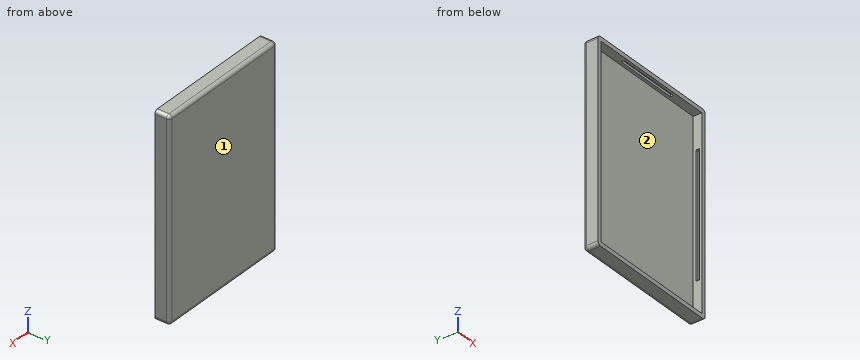
```python
from build123d import *

# Parameters (mm, degrees)
MAIN_LID_W          = 41.7
MAIN_LID_H          = 60.2
MAIN_LID_W_2        = 39.2
MAIN_LID_H_2        = 57.7
BOSS_EXTRUDE1_DEPTH = 4.5
MAIN_LID_3_W        = 39.2
MAIN_LID_3_H        = 57.7
CUT_EXTRUDE1_DEPTH  = 2.65
SKETCH2_W           = 17.05
SKETCH2_H           = 0.9
CUT_EXTRUDE2_DEPTH  = 0.75
SKETCH3_W           = 37.7
SKETCH3_H           = 1.05
CUT_EXTRUDE3_DEPTH  = 0.75
SKETCH4_W           = 19.2
SKETCH4_H           = 0.9
CUT_EXTRUDE4_DEPTH  = 0.75
FILLET1_R           = 1


with BuildPart() as part:
    # Main_Lid → Boss-Extrude1 (new body)
    # profile 1 of 2: a face of its own
    with BuildSketch(Plane(origin=(0, -69.305732589, 0), x_dir=(1, 0, 0), z_dir=(0, 1, 0))):
        with Locations((41.6, 0.1)):
            Rectangle(MAIN_LID_W, MAIN_LID_H)
        with Locations((41.6, 0.1)):
            Rectangle(MAIN_LID_W_2, MAIN_LID_H_2, mode=Mode.SUBTRACT)
    # profile 2 of 2: a face of its own
    with BuildSketch(Plane(origin=(0, -69.305732589, 0), x_dir=(1, 0, 0), z_dir=(0, 1, 0))):
        with Locations((41.6, 0.1)):
            Rectangle(MAIN_LID_W_2, MAIN_LID_H_2)
    extrude(amount=BOSS_EXTRUDE1_DEPTH)

    # Main_Lid_3 → Cut-Extrude1 (cut)
    with BuildSketch(Plane(origin=(0, -69.305732589, 0), x_dir=(1, 0, 0), z_dir=(0, 1, 0))):
        with Locations((41.6, 0.1)):
            Rectangle(MAIN_LID_3_W, MAIN_LID_3_H)
    extrude(amount=CUT_EXTRUDE1_DEPTH, mode=Mode.SUBTRACT)

    # Sketch2 → Cut-Extrude2 (cut)
    with BuildSketch(Plane.XY.offset(-28.95)):
        with Locations((49.675, -68.055732589)):
            Rectangle(SKETCH2_W, SKETCH2_H)
    extrude(amount=-CUT_EXTRUDE2_DEPTH, mode=Mode.SUBTRACT)

    # Sketch3 → Cut-Extrude3 (cut)
    with BuildSketch(Plane.ZY.offset(-61.2)):
        with Locations((-0.1, -67.980732589)):
            Rectangle(SKETCH3_W, SKETCH3_H)
    extrude(amount=-CUT_EXTRUDE3_DEPTH, mode=Mode.SUBTRACT)

    # Sketch4 → Cut-Extrude4 (cut)
    with BuildSketch(Plane(origin=(0, 0, 28.75), x_dir=(-1, 0, 0), z_dir=(0, 0, -1))):
        with Locations((-41.6, -68.055732589)):
            Rectangle(SKETCH4_W, SKETCH4_H)
    extrude(amount=-CUT_EXTRUDE4_DEPTH, mode=Mode.SUBTRACT)

    # Fillet1
    fillet1_edges = [part.edges().sort_by_distance(p)[0] for p in [
        (20.75, -67.055732589, 30),
        (41.6, -64.805732589, 30),
        (62.45, -64.805732589, -0.1),
        (41.6, -64.805732589, -30.2),
        (20.75, -64.805732589, -0.1),
        (20.75, -67.055732589, -30.2),
        (62.45, -67.055732589, -30.2),
        (62.45, -67.055732589, 30),
    ]]
    fillet(fillet1_edges, radius=FILLET1_R)


solid = part.part
```
Design review of the part built by this model. Coordinates are the model's own, in mm. Face numbers are marked on the shaded views. Coordinates: 2 decimals unless noted, no trailing zeros. Order: outer loops, then holes, each group sorted by start corner. A loop starts at its lowest first (then second) coordinate and runs counter-clockwise, first axis right, second up.
1) Take a section at B-B, the plane z = 3. Give the boundary of the cut face in (x, y).
2) Wall thickness on line 1 along Z through (x, y) = (60, -68.9); line 2 along X through (y, z) = (-67.6, -10); line 3 along X through (y, z) = (-66.7, 24.5): over which ranges is each line inside the solid? List them lowest first.
3) Clearance check with a flat-ended pin moving along its axis: pin 1 (4 mm diameter, centred on x = 32, z = -23.5, fed in from -Y). State where the tip first meets the part, or that it passes through.
4) Take a section at A-A, the plane x = 25. Give the boundary of the cut face in (y, z).
5) Take a section at C-C, the plane x = 42. Give the boundary of the cut face in (y, z), and give its area (3 significant figures).
6) Mouldability with a two-part tool opening along X and no side actions: class the marked faces 1 and 2 as +X half, -X half, draft (parallel to the pull), parting line (faces both ways), or undercut.
7) Take a section at D-D, the plane z = 25. Give the boundary of the cut face in (x, y).
Returned:
1. outline: (20.75, -69.31) - (22, -69.31) - (22, -66.66) - (61.2, -66.66) - (61.2, -67.46) - (61.95, -67.46) - (61.95, -68.51) - (61.2, -68.51) - (61.2, -69.31) - (62.45, -69.31) - (62.45, -65.81) arc R1 ccw to (61.45, -64.81) - (21.75, -64.81) arc R1 ccw to (20.75, -65.81) - close
2. line 1: z = -30.2 to -28.95, 28.75 to 30
2. line 2: x = 20.75 to 22, 61.95 to 62.45
2. line 3: x = 20.75 to 22, 61.2 to 62.45
3. pin 1: stops at y = -66.66
4. outline: (-69.31, -30.2) - (-65.81, -30.2) arc R1 ccw to (-64.81, -29.2) - (-64.81, 29) arc R1 ccw to (-65.81, 30) - (-69.31, 30) - (-69.31, 28.75) - (-66.66, 28.75) - (-66.66, -28.95) - (-69.31, -28.95) - close
5. outline: (-69.31, -30.2) - (-65.81, -30.2) arc R1 ccw to (-64.81, -29.2) - (-64.81, 29) arc R1 ccw to (-65.81, 30) - (-69.31, 30) - (-69.31, 28.75) - (-68.51, 28.75) - (-68.51, 29.5) - (-67.61, 29.5) - (-67.61, 28.75) - (-66.66, 28.75) - (-66.66, -28.95) - (-67.61, -28.95) - (-67.61, -29.7) - (-68.51, -29.7) - (-68.51, -28.95) - (-69.31, -28.95) - close
5. area: 116 mm2
6. face 1: draft
6. face 2: undercut
7. outline: (20.75, -69.31) - (22, -69.31) - (22, -66.66) - (61.2, -66.66) - (61.2, -69.31) - (62.45, -69.31) - (62.45, -65.81) arc R1 ccw to (61.45, -64.81) - (21.75, -64.81) arc R1 ccw to (20.75, -65.81) - close
